from build123d import *

# Parameters (mm, degrees)
F0_W     = 20
F0_H     = 25
F0_R     = 7.3
F1_DEPTH = 30
F3_DEPTH = 25
F5_DEPTH = 25.001
F6_W     = 20
F6_H     = 25
F7_DEPTH = 2


with BuildPart() as f1:
    # F0 (on Top) → F1 (new body)
    with BuildSketch(Plane.XY):
        Rectangle(F0_W, F0_H)
        Circle(F0_R, mode=Mode.SUBTRACT)
    extrude(amount=F1_DEPTH)

    # F2 (on face) → F3 (cut)
    with BuildSketch(Plane.YZ.offset(10)):
        with BuildLine():
            ThreePointArc((0, 7.1), (-1.1, 6), (0, 4.9))
            Line((0, 4.9), (0, 6))
            Line((0, 6), (0, 7.1))
        make_face()
        with BuildLine():
            ThreePointArc((1.1, 12), (-0.777817, 12.777817), (0, 10.9))
            ThreePointArc((0, 10.9), (0.777817, 11.222183), (1.1, 12))
        make_face()
        with BuildLine():
            Line((0, 6), (0, 4.9))
            ThreePointArc((0, 4.9), (0.777817, 5.222183), (1.1, 6))
            ThreePointArc((1.1, 6), (0.777817, 6.777817), (0, 7.1))
            Line((0, 7.1), (0, 6))
        make_face()
    extrude(amount=-F3_DEPTH, mode=Mode.SUBTRACT)

    # F4 (on face) → F5 (cut, through all)
    with BuildSketch(Plane(origin=(0, 12.5, 0), x_dir=(-1, 0, 0), z_dir=(0, 1, 0))):
        with BuildLine():
            ThreePointArc((0, 20.319805), (1.06066, 20.759145), (1.5, 21.819805))
            ThreePointArc((1.5, 21.819805), (-1.06066, 22.880465), (0, 20.319805))
        make_face()
    extrude(amount=-F5_DEPTH, mode=Mode.SUBTRACT)

    # F6 (on face) → F7 (join)
    with BuildSketch(Plane(origin=(0, 0, 0), x_dir=(1, 0, 0), z_dir=(0, 0, -1))):
        Rectangle(F6_W, F6_H)
    extrude(amount=F7_DEPTH)


solid = f1.part
For this review, take the finished solid that the model builds, in its own axes (mm). A direction names the side the tool comes from. Coordinates: 2 decimals unless noted, no trailing zeros. Order: outer loops, then holes, each group sorted by start corner. A loop starts at its lowest first (then second) coordinate and runs counter-clockwise, first axis right, second up. Notation, with made-up numbers: (-26, 35) - (24, 35) arc R29 ccw to (24, 68) - close; hole circle Ø2 at (38, 73.25). An arc over 180 degrees is marked (long way). Use one line per item in the form item = value.
Q1. Draft analysis for pull direction Y (two halves, no side actions). For faces 3 (the flat face through (0, 12.5, 14)), 4 (the flat face through (-10, 0, 14)), 5 (the flat face through (0, 0, 0)), 6 (the flat face through (0, -12.5, 14)), state which applies: +Y half, -Y half, draft (parallel to the pull), parting line (faces both ways), or undercut.
Checked values:
face_3 = +Y half
face_4 = draft
face_5 = undercut
face_6 = -Y half
Q2. For probe 1 along Y at (x, z) = (-8.8, 12); probe 2 along Y at (x, z) = (0, 9); probe 3 along X at (y, z) = (-2.75, 15.5), list the stretches that pass through material, from the lowest coordinate up. Write a range as from..to.
Checked values:
probe_1 = -12.5..-1.1, 1.1..12.5
probe_2 = -12.5..-7.3, 7.3..12.5
probe_3 = -10..-6.76, 6.76..10
Q3. Consider section C-C (x = -6.5). Give the boundary of the cut face in (y, z), then the cut area to 3 significant figures.
Checked values:
outline = (-12.5, -2) - (12.5, -2) - (12.5, 30) - (3.32, 30) - (3.32, 0) - (-3.32, 0) - (-3.32, 30) - (-12.5, 30) - close
area = 601 mm2
Q4. Consider section B-B (y = 2.5). Give the boundary of the cut face in (x, z), then the cut area to 3 significant figures.
Checked values:
outline = (-10, -2) - (10, -2) - (10, 30) - (6.86, 30) - (6.86, 0) - (-6.86, 0) - (-6.86, 30) - (-10, 30) - close
area = 228 mm2
Q5. Consider section A-A (z = 25). Give the boundary of the cut face in (x, y), then the cut area to 3 significant figures.
Checked values:
outline = (-10, -12.5) - (10, -12.5) - (10, 12.5) - (-10, 12.5) - close; hole circle Ø14.6 at (0, 0)
area = 333 mm2
Q6. For P1, Ø7.5, axis at x = 1, y = 2.5, coming from the +Z side, flat-tipped, find the tip position at first contact; note if it passes through.
Checked values:
P1 = 0
Q7. For faces 1 (the flat face through (10, 0, 14)), 2 (the cylindrical face through (6.74, -2.8, 14.79)), list the 3-axis set-ups (+Z, -Z, +X, -X, +Y, -Y) from which the entire face can be reached by the end or side of a thin tool; tool diameter is ignored.
Checked values:
face_1 = +Z, -Z, +X, +Y, -Y
face_2 = +Z
